Autodesk Inventor part; units mm, degrees
ref_plane "YZ Plane" through (0, 0, 0) normal (1, 0, 0) x (0, 1, 0)
ref_plane "XZ Plane" through (0, 0, 0) normal (0, 1, 0) x (-1, 0, 0)
ref_plane "XY Plane" through (0, 0, 0) normal (0, 0, 1) x (1, 0, 0)
sketch "Sketch1" plane through (0, 0, 0) normal (0, 1, 0) x (-1, 0, 0)
  circle A0 centre (0, 0) radius 55
  line L0 (0, 0) -> (15, 0)
  circle A1 centre (0, 0) radius 8 construction
  line L1 (0, 0) -> (21, 0)
  circle A2 centre (21, 0) radius 8 construction
  line L2 (0, 0) -> (42, 0)
  circle A3 centre (42, 0) radius 8 construction
  circle A4 centre (0, 0) radius 5
  circle A5 centre (21, 0) radius 5
  circle A6 centre (10.5, 18.1865) radius 5
  circle A7 centre (-10.5, 18.1865) radius 5
  circle A8 centre (-21, 0) radius 5
  circle A9 centre (-10.5, -18.1865) radius 5
  circle A10 centre (10.5, -18.1865) radius 5
  circle A11 centre (42, 0) radius 5
  circle A12 centre (36.3731, 21) radius 5
  circle A13 centre (21, 36.3731) radius 5
  circle A14 centre (0, 42) radius 5
  circle A15 centre (-21, 36.3731) radius 5
  circle A16 centre (-36.3731, 21) radius 5
  circle A17 centre (-42, 0) radius 5
  circle A18 centre (-36.3731, -21) radius 5
  circle A19 centre (-21, -36.3731) radius 5
  circle A20 centre (0, -42) radius 5
  circle A21 centre (21, -36.3731) radius 5
  circle A22 centre (36.3731, -21) radius 5
  dimension "d0" = 110
  dimension "d4" = 15
  dimension "d6" = 16
  dimension "d7" = 21
  dimension "d8" = 16
  dimension "d14" = 42
  dimension "d15" = 16
  dimension "d20" = 10
  dimension "d21" = 10
  dimension "d24" = 360
  dimension "d26" = 10
  dimension "d29" = 360
extrude "Extrusion1" add sketch "Sketch1" along normal blind 2
properties part number "separator_v2" material "Brass, Soft Yellow, Welded"
Part model, mm, in its own coordinate system. Round coordinates to 2 decimals unless told otherwise and drop trailing zeros. Order: outer loops, then holes, each group sorted by start corner. A loop starts at its lowest first (then second) coordinate and runs counter-clockwise, first axis right, second up. Notation, with made-up numbers: (-31.5, 41) -> (0.5, 41) arc R13 ccw to (0.5, 57) -> close; hole circle Ø10 at (79.5, -6.5). An arc over 180 degrees is marked (long way). Put each result on its own line as item: value.
Q1. Band-saw the part on D-D (z = -45.5). Give the cut face in (x, y).
From the geometry:
outline: (-30.9, 0) -> (-3.57, 0) -> (-3.57, 2) -> (-30.9, 2) -> close; (3.57, 0) -> (30.9, 0) -> (30.9, 2) -> (3.57, 2) -> close
Q2. Band-saw the part on B-B (z = -21). Give the cut face in (x, y).
From the geometry:
outline: (-50.83, 0) -> (-41.37, 0) -> (-41.37, 2) -> (-50.83, 2) -> close; (-31.37, 0) -> (-14.63, 0) -> (-14.63, 2) -> (-31.37, 2) -> close; (-6.37, 0) -> (6.37, 0) -> (6.37, 2) -> (-6.37, 2) -> close; (14.63, 0) -> (31.37, 0) -> (31.37, 2) -> (14.63, 2) -> close; (41.37, 0) -> (50.83, 0) -> (50.83, 2) -> (41.37, 2) -> close
Q3. Pin check, flat tip, straight feed: pin 1 Ø1 at (x, y) = (21, 0.5) entering from -Z. Stop position of the tip, or through.
From the geometry:
pin 1: stops at z = -51.04
Q4. Pull direction Z, two halves, no side cores. Call faces 1 (the face through (11.923, 0.986, 53.692)), 2 (the face through (5.88, 0.99, 20.1)), 3 (the face through (1, 2, -11)): pulls with the +Z half, pulls with the -Z half, needs draft (parallel to the pull), parting line crosses it, or undercut.
From the geometry:
face 1: parting line crosses it
face 2: undercut
face 3: needs draft
Q5. Band-saw the part on A-A (x = 0). Give the cut face in (y, z).
From the geometry:
outline: (0, -55) -> (2, -55) -> (2, -47) -> (0, -47) -> close; (0, -37) -> (2, -37) -> (2, -5) -> (0, -5) -> close; (0, 5) -> (2, 5) -> (2, 37) -> (0, 37) -> close; (0, 47) -> (2, 47) -> (2, 55) -> (0, 55) -> close
Q6. Band-saw the part on C-C (x = 34). Give the cut face in (y, z), and give its area (3 significant figures).
From the geometry:
outline: (0, -43.23) -> (2, -43.23) -> (2, -25.4) -> (0, -25.4) -> close; (0, -16.6) -> (2, -16.6) -> (2, 16.6) -> (0, 16.6) -> close; (0, 25.4) -> (2, 25.4) -> (2, 43.23) -> (0, 43.23) -> close
area: 138 mm2
Q7. Wall check: line 1 (Z direction, x = -0.5, y = 0.1); line 2 (X direction, y = 0.2, z = -19); line 3 (X direction, y = 0.6, z = 14). Give the ranges that are in metal, low to high. Write a range as [from, to].
From the geometry:
line 1: z = [-55, -46.97], [-37.03, -4.97], [4.97, 37.03], [46.97, 55]
line 2: x = [-51.61, -40.96], [-31.79, -15.43], [-5.57, 5.57], [15.43, 31.79], [40.96, 51.61]
line 3: x = [-53.19, -13.23], [-7.77, 7.77], [13.23, 53.19]
